Geometry check sheet. Reference: the model listing, model coordinates, mm. Face numbers are marked on the shaded views. Round coordinates to 2 decimals unless told otherwise and drop trailing zeros.
```python
from build123d import *

# Parameters (mm, degrees)
SKETCH2_W           = 30
SKETCH2_H           = 30
BOSS_EXTRUDE1_DEPTH = 50
SKETCH3_W           = 25
SKETCH3_H           = 25
CUT_EXTRUDE1_DEPTH  = 2.5
FILLET1_R           = 5


with BuildPart() as part:
    # Sketch2 → Boss-Extrude1 (new body)
    with BuildSketch(Plane(origin=(0, 0, 0), x_dir=(1, 0, 0), z_dir=(0, 1, 0))):
        Rectangle(SKETCH2_W, SKETCH2_H)
    extrude(amount=BOSS_EXTRUDE1_DEPTH)

    # Sketch3 → Cut-Extrude1 (cut)
    with BuildSketch(Plane(origin=(0, 50, 0), x_dir=(1, 0, 0), z_dir=(0, 1, 0))):
        Rectangle(SKETCH3_W, SKETCH3_H)
    extrude(amount=-CUT_EXTRUDE1_DEPTH, mode=Mode.SUBTRACT)

    # Fillet1
    fillet1_edges = [part.edges().sort_by_distance(p)[0] for p in [
        (15, 25, 15),
        (-15, 25, 15),
        (-15, 25, -15),
        (15, 25, -15),
    ]]
    fillet(fillet1_edges, radius=FILLET1_R)

    # Cut-Loft2: read off the stored shape, not the designer's step
    # Cut-Loft2: loft between two sections, ruled curve by curve
    cut_loft2_from = [
        Edge.make_bspline([(0, 0, -12.5), (-25, 0, -12.5), (-25, 0, 12.5), (0, 0, 12.5), (25, 0, 12.5), (25, 0, -12.5), (0, 0, -12.5)], [0, 0, 0, 0, 0.5, 0.5, 0.5, 1, 1, 1, 1], 3, [1, 0.333333333, 0.333333333, 1, 0.333333333, 0.333333333, 1]),
    ]
    cut_loft2_to = [
        Edge.make_bspline([(0.784484005, 47.5, -2.373728048), (-3.962972092, 47.5, -3.942696057), (-5.531940101, 47.5, 0.804760039), (-0.784484005, 47.5, 2.373728048), (3.962972092, 47.5, 3.942696057), (5.531940101, 47.5, -0.804760039), (0.784484005, 47.5, -2.373728048)], [0, 0, 0, 0, 0.5, 0.5, 0.5, 1, 1, 1, 1], 3, [1, 0.333333333, 0.333333333, 1, 0.333333333, 0.333333333, 1]),
    ]
    cut_loft2 = Solid(Shell([*[Face.make_surface_from_curves(cut_loft2_from[k], cut_loft2_to[k]) for k in range(1)], Face(Wire(cut_loft2_from)), Face(Wire(cut_loft2_to))]))
    add(cut_loft2, mode=Mode.SUBTRACT)


solid = part.part
```
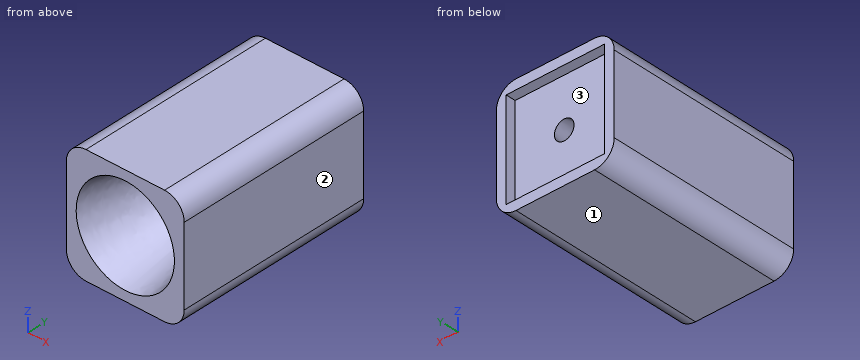
(1) Material ranges on line 1 (X direction, y = 25, z = -5.5); line 2 (X direction, y = 26, z = -5.5); line 3 (Z direction, x = 3, y = 42), recorded low to high.
Returned:
line 1: x = -15 to -4.62, 4.62 to 15
line 2: x = -15 to -4.28, 4.28 to 15
line 3: z = -15 to -2.01, 2.01 to 15
(2) Depth check by flat-ended pin: P1, Ø7.5, axis at x = 3, z = -5.5, coming from the +Y side. Enter the tip coordinate at first touch or a pass-through.
Returned:
P1: stops at y = 47.5
(3) Draft check along X on the marked faces 1, 2 and 3. Enter one of: released by +X, released by -X, zero draft, split by the parting line, or undercut.
Returned:
face 1: zero draft
face 2: released by +X
face 3: undercut
